Build history of the part. All positions in model axes, mm. A direction names the side the tool comes from. Round coordinates to 2 decimals unless told otherwise and drop trailing zeros. Order: outer loops, then holes, each group sorted by start corner. A loop starts at its lowest first (then second) coordinate and runs counter-clockwise, first axis right, second up. Notation, with made-up numbers: M 41,-33 L 85,-33 A37 cw 85,4 Z; hole C 49.25,-6.75 d8. An arc over 180 degrees is marked long. Use CSV: the item, a comma, the result in double quotes.
from build123d import *

# Parameters (mm, degrees)
SKETCH1_W           = 120
SKETCH1_H           = 10
BOSS_EXTRUDE1_DEPTH = 0.5
JACKS_R             = 1.75
BOSS_EXTRUDE2_DEPTH = 1
USB_PORT_W          = 1.8
USB_PORT_H          = 4
CUT_EXTRUDE2_DEPTH  = 0.2
LPATTERN1_COUNT     = 4
LPATTERN1_PITCH     = 2


with BuildPart() as part:
    # Sketch1 → Boss-Extrude1 (new body)
    with BuildSketch(Plane.XY):
        Rectangle(SKETCH1_W, SKETCH1_H)
    extrude(amount=BOSS_EXTRUDE1_DEPTH)

    # Jacks → Boss-Extrude2 (add)
    with BuildSketch(Plane.XY.offset(0.5)):
        with Locations(Location((23, -3, 0), (0, 0, 180))):
            Circle(JACKS_R)
        with Locations(Location((43, -3, 0), (0, 0, 180))):
            Circle(JACKS_R)
    extrude(amount=BOSS_EXTRUDE2_DEPTH)

    # usb port → Cut-Extrude2 (cut)
    with BuildSketch(Plane.XY.offset(0.5)):
        with Locations((-28.35, -3)):
            Rectangle(USB_PORT_W, USB_PORT_H)
    cut_extrude2 = extrude(amount=-CUT_EXTRUDE2_DEPTH, mode=Mode.SUBTRACT)

    # LPattern1: Cut-Extrude2 ×4
    with Locations(*[(i * LPATTERN1_PITCH, 0, 0) for i in range(1, LPATTERN1_COUNT)]):
        add(cut_extrude2, mode=Mode.SUBTRACT)


solid = part.part
(1) Two-plate mould, pull along X, no slides. Class faces 1 (the face through (-1, 0, 0)), 2 (the face through (41.383, -2.33, 0.993)): released by +X, released by -X, zero draft, split by the parting line, or undercut.
Answer block:
face 1,"zero draft"
face 2,"undercut"
(2) Cut at B-B, the plane x = 23. Give the cut face in (y, z).
Answer block:
outline,"M -5,0 L 5,0 L 5,0.5 L -1.25,0.5 L -1.25,1.5 L -4.75,1.5 L -4.75,0.5 L -5,0.5 Z"
(3) Drop flat-ended pins along their axis: pin 1 (0.5 mm diameter, centred on x = -28, y = -3.5, fed in from +Z); pin 2 (6 mm diameter, centred on x = -1, y = 1, fed in from +Z). Give the stop position or say it passes through.
Answer block:
pin 1,"stops at z = 0.3"
pin 2,"stops at z = 0.5"
(4) Wall check: line 1 (X direction, y = -2, z = 0.4); line 2 (X direction, y = -3.25, z = 0.65); line 3 (Z direction, x = -41, y = 2.5). Give the ranges that are in metal, low to high. Write a range as from..to.
Answer block:
line 1,"x = -60..-29.25, -27.45..-27.25, -25.45..-25.25, -23.45..-23.25, -21.45..60"
line 2,"x = 21.27..24.73, 41.27..44.73"
line 3,"z = 0..0.5"
(5) Cut at A-A, the plane y = -3. Give the cut face in (x, z), and give its area (3 significant figures).
Answer block:
outline,"M -60,0 L 60,0 L 60,0.5 L 44.75,0.5 L 44.75,1.5 L 41.25,1.5 L 41.25,0.5 L 24.75,0.5 L 24.75,1.5 L 21.25,1.5 L 21.25,0.5 L -21.45,0.5 L -21.45,0.3 L -23.25,0.3 L -23.25,0.5 L -23.45,0.5 L -23.45,0.3 L -25.25,0.3 L -25.25,0.5 L -25.45,0.5 L -25.45,0.3 L -27.25,0.3 L -27.25,0.5 L -27.45,0.5 L -27.45,0.3 L -29.25,0.3 L -29.25,0.5 L -60,0.5 Z"
area,"65.6 mm²"
(6) Tool access for faces 3 (the face through (43, -3, 1.5)), 4 (the face through (24.75, -3.08, 0.99)): list every direction of +Z, -Z, +X, -X, +Y, -Y with a clear straight run to the whole face (end or side of a thin tool).
Answer block:
face 3,"+Z, +X, -X, +Y, -Y"
face 4,"+Z"
(7) Cut at D-D, the plane y = 3.75. Give the cut face in (x, z).
Answer block:
outline,"M -60,0 L 60,0 L 60,0.5 L -60,0.5 Z"
(8) Cut at C-C, the plane z = 0.9. Give the cut face in (x, y).
Answer block:
outline,"C 23,-3 d3.5; C 43,-3 d3.5"
